```python
from build123d import *

# Parameters (mm, degrees)
EXTRUDE_2_DEPTH           = 35
SKETCH_3_W                = 9.6
SKETCH_3_H                = 9.6
EXTRUDE_3_DEPTH           = 35
SKETCH_8_W                = 10
SKETCH_8_H                = 6.4
EXTRUDE_4_DEPTH           = 35
EXTRUDE_5_DEPTH           = 2
FILLET_1_R                = 2
SKETCH_11_R               = 1.45
CUT_EXTRUDE_7_DEPTH       = 8
CUT_EXTRUDE_17_DEPTH      = 1.6
SKETCH_77_W               = 0.9
SKETCH_77_H               = 3.100006964
SKETCH_77_H_2             = 1.824993516
SKETCH_77_H_3             = 8.175815104
EXTRUDE_15_DEPTH          = 2
SKETCH_78_W               = 0.9
SKETCH_78_H               = 1.824993516
SKETCH_78_H_2             = 8.175815104
SKETCH_78_H_3             = 3.100006964
CUT_EXTRUDE_20_DEPTH      = 2
SKETCH_79_W               = 3.100006964
SKETCH_79_H               = 0.2
SKETCH_79_W_2             = 1.824993516
SKETCH_79_W_3             = 8.175815104
CUT_EXTRUDE_21_DEPTH      = 0.7
CUT_EXTRUDE_18_DEPTH      = 4.5
SKETCH_32_W               = 113.6
SKETCH_32_H               = 166.2
EXTRUDE_6_DEPTH           = 1.6
SKETCH_33_W               = 7
SKETCH_33_H               = 150.2
CUT_EXTRUDE_19_DEPTH      = 1.6
SKETCH_35_R               = 3.65
EXTRUDE_7_DEPTH           = 5
HOLE_WIZARD_3_D           = 5.3
HOLE_WIZARD_3_CSINK_D     = 6.3
HOLE_WIZARD_3_CSINK_ANGLE = 90
SKETCH_48_R               = 3.65
EXTRUDE_8_DEPTH           = 5
SKETCH_53_R               = 3.65
EXTRUDE_9_DEPTH           = 5
SKETCH_59_R               = 3.65
EXTRUDE_12_DEPTH          = 5
SKETCH_64_R               = 3.65
EXTRUDE_13_DEPTH          = 5
SKETCH_72_R               = 3.65
EXTRUDE_14_DEPTH          = 5
HOLE_WIZARD_5_D           = 5.3
HOLE_WIZARD_5_CSINK_D     = 6.3
HOLE_WIZARD_5_CSINK_ANGLE = 90
FILLET_2_R                = 1
SKETCH_81_W               = 10
SKETCH_81_H               = 163
EXTRUDE_16_DEPTH          = 6


with BuildPart() as part:
    # Эскиз2 → Бобышка-Вытянуть2 (new body)
    with BuildSketch(Plane.XZ):
        Polygon((-54.2, 83.1), (54.2, 83.1), (54.2, -83.1), (-54.2, -83.1), (-59.4, -83.1), (-59.4, -81.5), (-54.2, -81.5), (52.6, -81.5), (52.6, 81.5), (-54.2, 81.5), (-59.4, 81.5), (-59.4, 83.1), align=None)
    extrude(amount=EXTRUDE_2_DEPTH)

    # Эскиз3 → Бобышка-Вытянуть3 (add)
    with BuildSketch(Plane.XZ):
        with Locations((47.8, 76.7)):
            Rectangle(SKETCH_3_W, SKETCH_3_H)
        with Locations((47.8, -76.7)):
            Rectangle(SKETCH_3_W, SKETCH_3_H)
    extrude(amount=EXTRUDE_3_DEPTH)

    # Эскиз8 → Бобышка-Вытянуть4 (add)
    with BuildSketch(Plane.XZ):
        with Locations((-54.4, 78.3)):
            Rectangle(SKETCH_8_W, SKETCH_8_H)
    extrude_4 = extrude(amount=EXTRUDE_4_DEPTH)

    # Зеркальное отражение1: Бобышка-Вытянуть4 across plane
    add(extrude_4.mirror(Plane.XY))

    # Эскиз10 → Бобышка-Вытянуть5 (add)
    with BuildSketch(Plane.XZ.offset(35)):
        Polygon((-59.4, 83.1), (-59.4, 75.1), (-58.7, 75.1), (-58.7, 82.4), (53.5, 82.4), (53.5, -82.4), (-58.7, -82.4), (-58.7, -75.1), (-59.4, -75.1), (-59.4, -83.1), (54.2, -83.1), (54.2, 83.1), align=None)
    extrude(amount=EXTRUDE_5_DEPTH)

    # Эскиз69 → Отверстие2 (revolve, cut)
    with BuildSketch(Plane(origin=(-53.9, -25, -83.1), x_dir=(0, 1, 0), z_dir=(1, 0, 0))):
        Polygon((0, 0), (0, 9), (1.55, 9), (1.55, 4.45), (3, 3), (3, 0), align=None)
    hole_wizard_2 = revolve(axis=Axis((-53.9, -25, -89.230023899), (0, 0, 1)), mode=Mode.SUBTRACT)

    # Зеркальное отражение2: Отверстие2 across plane
    add(hole_wizard_2.mirror(Plane.XY), mode=Mode.SUBTRACT)

    # Скругление1
    fillet_1_edges = [part.edges().sort_by_distance(p)[0] for p in [
        (43, -17.5, 71.9),
        (43, -17.5, -71.9),
    ]]
    fillet(fillet_1_edges, radius=FILLET_1_R)

    # Эскиз11 → Вырез-Вытянуть7 (cut)
    with BuildSketch(Plane.XZ.offset(35)):
        with Locations((47.8, 76.7)):
            Circle(SKETCH_11_R)
        with Locations((47.8, -76.7)):
            Circle(SKETCH_11_R)
    extrude(amount=-CUT_EXTRUDE_7_DEPTH, mode=Mode.SUBTRACT)

    # Эскиз24 → Вырез-Вытянуть17 (cut)
    with BuildSketch(Plane(origin=(54.2, 0, 0), x_dir=(0, 0, -1), z_dir=(1, 0, 0))):
        Polygon((-67.115753945, -24.45856124), (-54.915753678, -24.45856124), (-54.900002552, -24.45856124), (-54.900002552, -37), (-54.950002552, -37), (-67.200003552, -37), (-67.200003552, -24.45856124), align=None)
        with BuildLine():
            Line((26.600813792, -24.458561201), (26.600813792, -37))
            Line((26.600813792, -37), (63.100006082, -37))
            Line((63.100006082, -37), (63.100006082, -24.458561201))
            Line((63.100006082, -24.458561201), (60.600006082, -24.458561201))
            Line((60.600006082, -24.458561201), (60.600006082, -13.958561201))
            ThreePointArc((60.600006082, -13.958561201), (58.686114673, -9.338018606), (54.065572078, -7.424127197))
            Line((54.065572078, -7.424127197), (35.635247795, -7.424127197))
            ThreePointArc((35.635247795, -7.424127197), (31.0147052, -9.338018606), (29.100813792, -13.958561201))
            Line((29.100813792, -13.958561201), (29.100813792, -24.458561201))
            Line((29.100813792, -24.458561201), (26.600813792, -24.458561201))
        make_face()
        Polygon((-33.275002252, -37), (18.424998688, -37), (18.424998688, -28.5), (14.924998688, -28.5), (14.924998688, -26.5), (12.424998688, -26.5), (12.424998688, -28.5), (-5.875001312, -28.5), (-5.875001312, -26.5), (-8.975002252, -26.5), (-8.975002252, -28.5), (-27.275002252, -28.5), (-27.275002252, -26.5), (-29.775002252, -26.5), (-29.775002252, -28.5), (-33.275002252, -28.5), align=None)
        Polygon((-51.799995588, -37), (-35.099995768, -37), (-35.099995768, -28.5), (-38.601386518, -28.5), (-38.601386518, -26.5), (-41.101386518, -26.5), (-41.101386518, -28.5), (-45.799995588, -28.5), (-45.799995588, -26.5), (-48.299995588, -26.5), (-48.299995588, -28.5), (-51.799995588, -28.5), align=None)
    extrude(amount=-CUT_EXTRUDE_17_DEPTH, mode=Mode.SUBTRACT)

    # Эскиз77 → Бобышка-Вытянуть15 (add)
    with BuildSketch(Plane.XZ.offset(35)):
        with Locations((53.05, 53.34999907)):
            Rectangle(SKETCH_77_W, SKETCH_77_H)
        with Locations((53.05, 34.18749901)):
            Rectangle(SKETCH_77_W, SKETCH_77_H_2)
        with Locations((53.05, -22.51290624)):
            Rectangle(SKETCH_77_W, SKETCH_77_H_3)
    extrude(amount=EXTRUDE_15_DEPTH)

    # Эскиз78 → Вырез-Вытянуть20 (cut)
    with BuildSketch(Plane.XZ.offset(37)):
        with Locations((53.75, 34.18749901)):
            Rectangle(SKETCH_78_W, SKETCH_78_H)
        with Locations((53.75, -22.51290624)):
            Rectangle(SKETCH_78_W, SKETCH_78_H_2)
        with Locations((53.75, 53.34999907)):
            Rectangle(SKETCH_78_W, SKETCH_78_H_3)
    extrude(amount=-CUT_EXTRUDE_20_DEPTH, mode=Mode.SUBTRACT)

    # Эскиз79 → Вырез-Вытянуть21 (cut)
    with BuildSketch(Plane(origin=(53.3, 0, 0), x_dir=(0, 0, -1), z_dir=(1, 0, 0))):
        with Locations((-53.34999907, -36.9)):
            Rectangle(SKETCH_79_W, SKETCH_79_H)
        with Locations((-34.18749901, -36.9)):
            Rectangle(SKETCH_79_W_2, SKETCH_79_H)
        with Locations((22.51290624, -36.9)):
            Rectangle(SKETCH_79_W_3, SKETCH_79_H)
    extrude(amount=-CUT_EXTRUDE_21_DEPTH, mode=Mode.SUBTRACT)

    # Эскиз1 → Вырез-Вытянуть18 (cut)
    with BuildSketch(Plane(origin=(0, 0, 0), x_dir=(1, 0, 0), z_dir=(0, 1, 0))):
        Polygon((-54.2, 83.1), (-61.2, 83.1), (-61.2, -83.1), (-54.2, -83.1), (54.2, -83.1), (54.2, 83.1), align=None)
    extrude(amount=-CUT_EXTRUDE_18_DEPTH, mode=Mode.SUBTRACT)

    # Эскиз32 → Бобышка-Вытянуть6 (add)
    with BuildSketch(Plane(origin=(0, -4.5, 0), x_dir=(1, 0, 0), z_dir=(0, 1, 0))):
        with Locations((-2.6, 0)):
            Rectangle(SKETCH_32_W, SKETCH_32_H)
    extrude(amount=EXTRUDE_6_DEPTH)

    # Эскиз33 → Вырез-Вытянуть19 (cut)
    with BuildSketch(Plane(origin=(0, -2.9, 0), x_dir=(1, 0, 0), z_dir=(0, 1, 0))):
        with Locations((-57.7, 0)):
            Rectangle(SKETCH_33_W, SKETCH_33_H)
    extrude(amount=-CUT_EXTRUDE_19_DEPTH, mode=Mode.SUBTRACT)

    # Эскиз35 → Бобышка-Вытянуть7 (add)
    with BuildSketch(Plane.XZ.offset(4.5)):
        with Locations((5.169259644, 49.00012207)):
            Circle(SKETCH_35_R)
    extrude(amount=EXTRUDE_7_DEPTH)

    # Отверстие3 (through all)
    with Locations(Plane(origin=(0, -9.5, 0), x_dir=(-1, 0, 0), z_dir=(0, -1, 0))):
        with Locations((-5.169259644, -49.00012207)):
            CounterSinkHole(HOLE_WIZARD_3_D / 2, HOLE_WIZARD_3_CSINK_D / 2, counter_sink_angle=HOLE_WIZARD_3_CSINK_ANGLE)

    # Эскиз48 → Бобышка-Вытянуть8 (add)
    with BuildSketch(Plane.XZ.offset(4.5)):
        with Locations((-18.21427002, -53.725112916)):
            Circle(SKETCH_48_R)
    extrude(amount=EXTRUDE_8_DEPTH)

    # Эскиз53 → Бобышка-Вытянуть9 (add)
    with BuildSketch(Plane.XZ.offset(4.5)):
        with Locations((16.144265744, 49.00012207)):
            Circle(SKETCH_53_R)
    extrude(amount=EXTRUDE_9_DEPTH)

    # Эскиз59 → Бобышка-Вытянуть12 (add)
    with BuildSketch(Plane.XZ.offset(4.5)):
        with Locations((-10.9749991, -53.725112916)):
            Circle(SKETCH_59_R)
    extrude(amount=EXTRUDE_12_DEPTH)

    # Эскиз64 → Бобышка-Вытянуть13 (add)
    with BuildSketch(Plane.XZ.offset(4.5)):
        with Locations((5.172398423, 58.982823693)):
            Circle(SKETCH_64_R)
    extrude(amount=EXTRUDE_13_DEPTH)

    # Эскиз72 → Бобышка-Вытянуть14 (add)
    with BuildSketch(Plane.XZ.offset(4.5)):
        with Locations((16.144265744, 58.982823693)):
            Circle(SKETCH_72_R)
    extrude(amount=EXTRUDE_14_DEPTH)

    # Отверстие5 (through all)
    with Locations(Plane(origin=(0, -9.5, 0), x_dir=(-1, 0, 0), z_dir=(0, -1, 0))):
        with Locations((-16.144265744, -58.982823693), (-16.144265744, -49.00012207), (-5.172398423, -58.982823693), (10.9749991, 53.725112916), (18.21427002, 53.725112916)):
            CounterSinkHole(HOLE_WIZARD_5_D / 2, HOLE_WIZARD_5_CSINK_D / 2, counter_sink_angle=HOLE_WIZARD_5_CSINK_ANGLE)

    # Скругление2
    fillet_2_edges = [part.edges().sort_by_distance(p)[0] for p in [
        (54.2, -19.95, 83.1),
        (54.2, -19.95, -83.1),
        (-59.4, -19.95, -83.1),
        (-59.4, -19.95, 83.1),
        (-2.6, -2.9, 83.1),
        (54.2, -2.9, 0),
        (-2.6, -2.9, -83.1),
        (-59.4, -2.9, -79.1),
        (-59.4, -2.9, 79.1),
    ]]
    fillet(fillet_2_edges, radius=FILLET_2_R)

    # Эскиз81 → Бобышка-Вытянуть16 (add)
    with BuildSketch(Plane.XZ.offset(4.5)):
        with Locations((27.6, 0)):
            Rectangle(SKETCH_81_W, SKETCH_81_H)
        with Locations((-44.4, 0)):
            Rectangle(SKETCH_81_W, SKETCH_81_H)
    extrude(amount=EXTRUDE_16_DEPTH)


solid = part.part
```
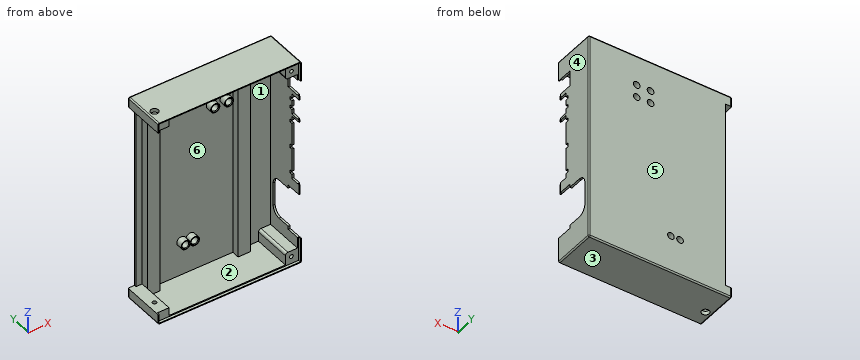
Design review of the part built by this model. Coordinates are the model's own, in mm. Face numbers are marked on the shaded views. A direction names the side the tool comes from. Coordinates: 2 decimals unless noted, no trailing zeros. Order: outer loops, then holes, each group sorted by start corner. A loop starts at its lowest first (then second) coordinate and runs counter-clockwise, first axis right, second up. Notation, with made-up numbers: M 85.5,26 L 99.5,26 A26 ccw 99.5,51 Z; hole C 8,79.25 d6. An arc over 180 degrees is marked long. Answer as a JSON object with one key per item and string values. Group by question number.
1) For pin 1 (2 mm diameter, centred on x = -8, z = 57.5, fed in from -Y); pin 2 (0.5 mm diameter, centred on x = 53.5, y = -32.5, fed in from -Z); pin 3 (5.5 mm diameter, centred on x = -53.9, y = -25, fed in from -Z); pin 4 (0.5 mm diameter, centred on x = 54, y = -28, fed in from +Z), all flat-tipped, find the tip position at first contact; note any pin that passes through.
2) Mouldability with a two-part tool opening along Z and no side actions: class the marked faces 1, 2, 3 and 4 as pulls with the +Z half, pulls with the -Z half, needs draft (parallel to the pull), parting line crosses it, or undercut.
3) Add section D-D, the plane z = -31. Write out the cut boundary in (x, y), then the cut area to 3 significant figures.
4) Add section B-B, the plane x = -26. Write out the cut boundary in (y, z).
5) Add section C-C, the plane z = -66. Write out the cut boundary in (x, y).
6) Tool access review of the marked faces 5 and 6: name each direction out of +Z, -Z, +X, -X, +Y, -Y from which nothing blocks a thin tool from reaching the whole face with its end or side.
7) Wall thickness on L1, parallel to X at y = -25, z = -76.6; L2, parallel to X at y = -6, z = -42.5; L3, parallel to Z at x = 47.8, y = -30.5: over which ranges is each line inside the solid? List them lowest first.
8) Add section A-A, the plane y = -18.5. Write out the cut boundary in (x, z), then the cut area to 3 significant figures.
Computed values:
{
 "1": {"pin 1": "stops at y = -4.5", "pin 2": "stops at z = -83.1", "pin 3": "stops at z = -79.85", "pin 4": "stops at z = 82.94"},
 "2": {"face 1": "undercut", "face 2": "undercut", "face 3": "pulls with the -Z half", "face 4": "needs draft"},
 "3": {"outline": "M -54.2,-4.5 L -49.4,-4.5 L -49.4,-10.5 L -39.4,-10.5 L -39.4,-4.5 L 22.6,-4.5 L 22.6,-10.5 L 32.6,-10.5 L 32.6,-4.5 L 52.6,-4.5 L 52.6,-9.35 L 54.2,-9.35 L 54.2,-3.9 A1 ccw 53.2,-2.9 L -54.2,-2.9 Z", "area": "301 mm^2"},
 "4": {"outline": "M -37,-83.1 L -3.9,-83.1 A1 ccw -2.9,-82.1 L -2.9,82.1 A1 ccw -3.9,83.1 L -37,83.1 L -37,82.4 L -35,82.4 L -35,81.5 L -4.5,81.5 L -4.5,-81.5 L -35,-81.5 L -35,-82.4 L -37,-82.4 Z"},
 "5": {"outline": "M -54.2,-4.5 L -49.4,-4.5 L -49.4,-10.5 L -39.4,-10.5 L -39.4,-4.5 L 22.6,-4.5 L 22.6,-10.5 L 32.6,-10.5 L 32.6,-4.5 L 52.6,-4.5 L 52.6,-35 L 53.5,-35 L 53.5,-37 L 54.2,-37 L 54.2,-3.9 A1 ccw 53.2,-2.9 L -54.2,-2.9 Z"},
 "6": {"face 5": "+Z, -Z, +X, -X, +Y", "face 6": "-Y"},
 "7": {"L1": "x = -59.4 to -55.45, -52.35 to -49.4, 43 to 54.2", "L2": "x = -49.4 to -39.4, 22.6 to 32.6, 52.6 to 54.2", "L3": "z = -83.1 to -78.15, -75.25 to -71.9, 71.9 to 75.25, 78.15 to 83.1"},
 "8": {"outline": "M -59.4,-82.1 A1 ccw -58.4,-83.1 L 53.2,-83.1 A1 ccw 54.2,-82.1 L 54.2,-60.6 L 52.6,-60.6 L 52.6,-71.9 L 45,-71.9 A2 ccw 43,-73.9 L 43,-81.5 L -49.4,-81.5 L -49.4,-75.1 L -59.4,-75.1 Z; M -59.4,75.1 L -49.4,75.1 L -49.4,81.5 L 43,81.5 L 43,73.9 A2 ccw 45,71.9 L 52.6,71.9 L 52.6,-29.1 L 54.2,-29.1 L 54.2,82.1 A1 ccw 53.2,83.1 L -58.4,83.1 A1 ccw -59.4,82.1 Z", "area": "884 mm^2"}
}
